For this review, take the finished solid that the model builds, in its own axes (mm). Give positions to 0.01 mm unless a question says otherwise; leave off trailing zeros. Loops run counter-clockwise (first coordinate to the right, second up) from the corner with the lowest first, then second, coordinate; pieces in that order, holes last. Notation, with made-up numbers: (-2, 66.5) - (34, 66.5) arc R6 cw to (34, 73.5) - close; hole circle Ø1 at (59.5, 53.25). An arc over 180 degrees is marked (long way). Answer in a Markdown table with one row per item.
```python
from build123d import *

# Parameters (mm, degrees)
SKETCH1_R           = 2.75
BOSS_EXTRUDE1_DEPTH = 2
FILLET1_R           = 1


with BuildPart() as part:
    # Sketch1 → Boss-Extrude1 (new, symmetric)
    with BuildSketch(Plane.XY):
        Polygon((0, 0), (0, 79), (39, 79), (79, 39), (79, 0), align=None)
        with Locations((9.5, 9.5)):
            Circle(SKETCH1_R, mode=Mode.SUBTRACT)
        with Locations((29.5, 9.5)):
            Circle(SKETCH1_R, mode=Mode.SUBTRACT)
        with Locations((49.5, 9.5)):
            Circle(SKETCH1_R, mode=Mode.SUBTRACT)
        with Locations((9.5, 29.5)):
            Circle(SKETCH1_R, mode=Mode.SUBTRACT)
        with Locations((9.5, 49.5)):
            Circle(SKETCH1_R, mode=Mode.SUBTRACT)
        with Locations((69.5, 9.5)):
            Circle(SKETCH1_R, mode=Mode.SUBTRACT)
        with Locations((69.5, 29.5)):
            Circle(SKETCH1_R, mode=Mode.SUBTRACT)
        with Locations((49.5, 29.5)):
            Circle(SKETCH1_R, mode=Mode.SUBTRACT)
        with Locations((29.5, 29.5)):
            Circle(SKETCH1_R, mode=Mode.SUBTRACT)
        with Locations((29.5, 49.5)):
            Circle(SKETCH1_R, mode=Mode.SUBTRACT)
        with Locations((29.5, 69.5)):
            Circle(SKETCH1_R, mode=Mode.SUBTRACT)
        with Locations((9.5, 69.5)):
            Circle(SKETCH1_R, mode=Mode.SUBTRACT)
    extrude(amount=BOSS_EXTRUDE1_DEPTH, both=True)

    # Fillet1
    fillet1_edges = [part.edges().sort_by_distance(p)[0] for p in [
        (59, 59, 2),
        (19.5, 79, 2),
        (0, 39.5, 2),
        (39.5, 0, 2),
        (79, 19.5, 2),
        (0, 0, 0),
        (0, 79, 0),
        (39, 79, 0),
        (79, 39, 0),
        (79, 0, 0),
    ]]
    fillet(fillet1_edges, radius=FILLET1_R)


solid = part.part
```
1. Wall thickness on line 1 (Y direction, x = 29.5, z = -0.85); line 2 (X direction, y = 28, z = -0.9): over which ranges is each line inside the solid? List them lowest first. Write a range as [from, to].
Values:
| item | result |
|---|---|
| line 1 | y = [0, 6.75], [12.25, 26.75], [32.25, 46.75], [52.25, 66.75], [72.25, 79] |
| line 2 | x = [0, 7.2], [11.8, 27.2], [31.8, 47.2], [51.8, 67.2], [71.8, 79] |
2. Mouldability with a two-part tool opening along Y and no side actions: class faces 1 (the face through (40, 0, 0)), 2 (the face through (40, 40, -2)), 3 (the face through (66.753, 9.621, -0.028)), 4 (the face through (20, 79, 0)) as released by +Y, released by -Y, zero draft, split by the parting line, or undercut.
Values:
| item | result |
|---|---|
| face 1 | released by -Y |
| face 2 | zero draft |
| face 3 | undercut |
| face 4 | released by +Y |
3. We need section C-C, the plane x = 49. Count the separate pieces of the cut face and the enclosed holes in it, and give its area (3 significant figures).
Values:
| item | result |
|---|---|
| separate pieces | 3 |
| enclosed holes | 0 |
| area | 232 mm^2 |
4. Clearance check with a flat-ended pin moving along its axis: pin 1 (3.5 mm diameter, centred on x = 29.5, y = 9.5, fed in from -Z). State where the tip first meets the part, or that it passes through.
Values:
| item | result |
|---|---|
| pin 1 | passes through |
5. We need section A-A, the plane x = 9.5. Give the boundary of the cut face in (y, z), and give its area (3 significant figures).
Values:
| item | result |
|---|---|
| outline | (0, -2) - (6.75, -2) - (6.75, 2) - (1, 2) arc R1 ccw to (0, 1) - close; (12.25, -2) - (26.75, -2) - (26.75, 2) - (12.25, 2) - close; (32.25, -2) - (46.75, -2) - (46.75, 2) - (32.25, 2) - close; (52.25, -2) - (66.75, -2) - (66.75, 2) - (52.25, 2) - close; (72.25, -2) - (79, -2) - (79, 1) arc R1 ccw to (78, 2) - (72.25, 2) - close |
| area | 228 mm^2 |
